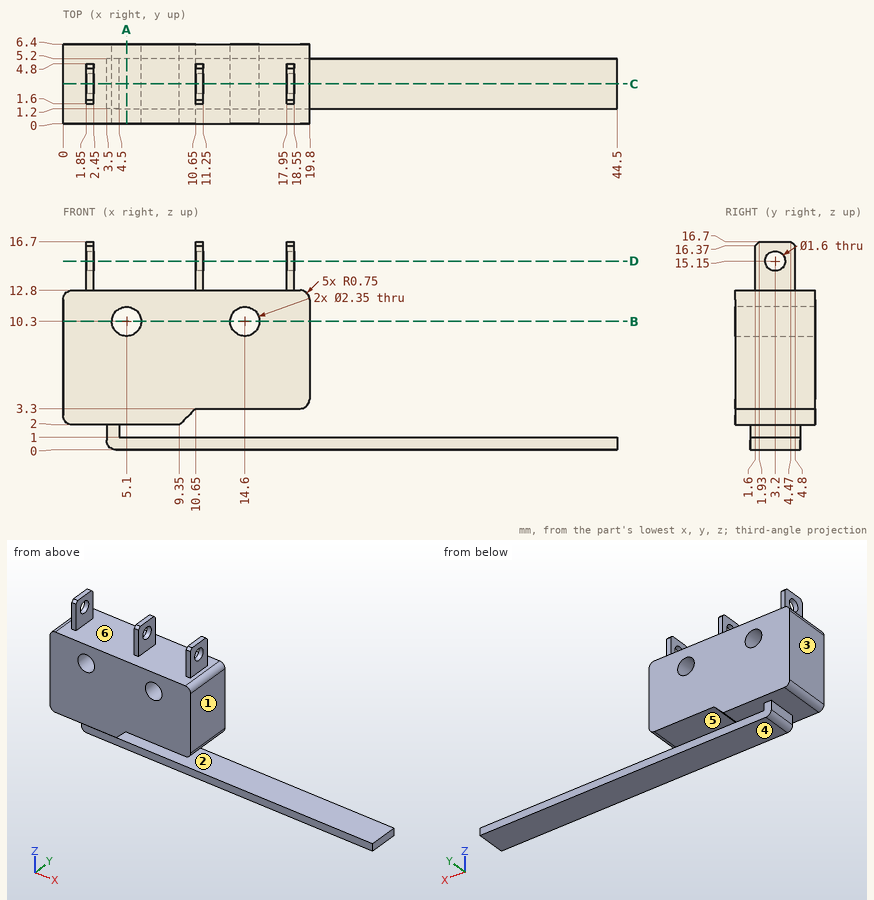
Drawing for the job (mm, zero at the part's lowest x, y, z). A direction names the side the tool comes from. Coordinates: 2 decimals unless noted, no trailing zeros. Write each loop counter-clockwise with the first axis right and the second up, starting at its lowest first coordinate (ties: lowest second). Pieces come first, ordered by that corner, then holes. Notation, with made-up numbers: (70.5, -7) -> (101.5, -7) arc R32 cw to (101.5, 31) -> close; hole circle Ø1 at (89.5, 5). An arc over 180 degrees is marked (long way). One line per item, written item: value. Start each with the question number.
1) Probe probe 1 along X at (y, z) = (4.75, 10.3) (3 decimals); probe 2 along X at (y, z) = (2.75, 14); probe 3 along Y at (x, z) = (2.2, 15.15). List the from-to ranges inside material, lowest first.
2) Pull direction Z, two halves, no side cores. Call the marked faces 4, 5 and 6: +Z half, -Z half, draft (parallel to the pull), parting line (faces both ways), or undercut.
3) Slice it at A-A on x = 5.1. Write the cut outline in (y, z) (3 decimals), then the cut area to 3 significant figures.
4) Slice it at C-C on y = 3.2. Count the separate pieces of the cut face and the enclosed holes in it, then the cut area to 3 significant figures.
5) Flat gauge pins, fed straight in: pin 1 Ø2 at (y, z) = (3, 8) entering from +X; pin 2 Ø0.5 at (x, z) = (2, 14.5) entering from +Y; pin 3 Ø3.5 at (y, z) = (3, 15.5) entering from -X. Where does each tip first touch, or does it go through?
6) Which spindle directions (+Z, -Z, +X, -X, +Y, -Y) get a long thin tool onto all of the face, cutting with end or side? Do the marked faces 1, 2 and 3. Say none if no direction does.
7) Slice it at D-D on z = 15.15. Write the cut outline in (x, y), then the cut area to 3 significant figures.
8) Slice it at B-B on z = 10.3. Write the cut outline in (x, y) (3 decimals).
Answers follow:
1. probe 1: 0 to 3.925, 6.275 to 13.425, 15.775 to 19.8
1. probe 2: 1.85 to 2.45, 10.65 to 11.25, 17.95 to 18.55
1. probe 3: 1.6 to 2.4, 4 to 4.8
2. face 4: -Z half
2. face 5: undercut
2. face 6: +Z half
3. outline: (0, 2) -> (6.4, 2) -> (6.4, 9.125) -> (0, 9.125) -> close; (0, 11.475) -> (6.4, 11.475) -> (6.4, 12.8) -> (0, 12.8) -> close; (1.2, 0) -> (5.2, 0) -> (5.2, 1) -> (1.2, 1) -> close
3. area: 58.1 mm2
4. separate pieces: 4
4. enclosed holes: 2
4. area: 238 mm2
5. pin 1: x = 19.8
5. pin 2: y = 4.8
5. pin 3: x = 1.85
6. face 1: +Z, +X, +Y, -Y
6. face 2: +X, +Y, -Y
6. face 3: +Z, -Z, -X, +Y, -Y
7. outline: (1.85, 1.6) -> (2.45, 1.6) -> (2.45, 2.4) -> (1.85, 2.4) -> close; (1.85, 4) -> (2.45, 4) -> (2.45, 4.8) -> (1.85, 4.8) -> close; (10.65, 1.6) -> (11.25, 1.6) -> (11.25, 2.4) -> (10.65, 2.4) -> close; (10.65, 4) -> (11.25, 4) -> (11.25, 4.8) -> (10.65, 4.8) -> close; (17.95, 1.6) -> (18.55, 1.6) -> (18.55, 2.4) -> (17.95, 2.4) -> close; (17.95, 4) -> (18.55, 4) -> (18.55, 4.8) -> (17.95, 4.8) -> close
7. area: 2.88 mm2
8. outline: (0, 0) -> (3.925, 0) -> (3.925, 6.4) -> (0, 6.4) -> close; (6.275, 0) -> (13.425, 0) -> (13.425, 6.4) -> (6.275, 6.4) -> close; (15.775, 0) -> (19.8, 0) -> (19.8, 6.4) -> (15.775, 6.4) -> close
